```python
from build123d import *

# Parameters (mm, degrees)
F0_W     = 609.6
F0_H     = 304.8
F1_DEPTH = 19.05
F2_W     = 10.795
F2_H     = 52.07
F3_DEPTH = 38.101
F4_W     = 127
F4_H     = 177.8
F5_DEPTH = 6.35


with BuildPart() as f1:
    # F0 (on Top) → F1 (new body, symmetric)
    with BuildSketch(Plane.XY):
        Rectangle(F0_W, F0_H)
    extrude(amount=F1_DEPTH, both=True)

    # F2 (on face) → F3 (cut, through all)
    with BuildSketch(Plane.XY.offset(19.05)):
        with Locations((-152.4, 0)):
            Rectangle(F2_W, F2_H)
        with Locations((152.4, 0)):
            Rectangle(F2_W, F2_H)
    extrude(amount=-F3_DEPTH, mode=Mode.SUBTRACT)

    # F4 (on face) → F5 (cut)
    with BuildSketch(Plane(origin=(0, 0, -19.05), x_dir=(1, 0, 0), z_dir=(0, 0, -1))):
        with Locations((-152.4, 0)):
            Rectangle(F4_W, F4_H)
        with Locations((152.4, 0)):
            Rectangle(F4_W, F4_H)
    extrude(amount=-F5_DEPTH, mode=Mode.SUBTRACT)


solid = f1.part
```
Build history of the part. All positions in model axes, mm. A direction names the side the tool comes from. Give positions to 0.01 mm unless a question says otherwise; leave off trailing zeros. Loops run counter-clockwise (first coordinate to the right, second up) from the corner with the lowest first, then second, coordinate; pieces in that order, holes last.
1) 3-axis set-ups, long thin cutter, end or side, ignore diameter. For faces 4 (the face through (-4, 152.4, 0)), 5 (the face through (-167, -1, -12.7)), 6 (the face through (147.002, 0, 3)): which of +Z, -Z, +X, -X, +Y, -Y reach the whole face in a straight line?
Values follow:
face 4: +Z, -Z, +X, -X, +Y
face 5: -Z
face 6: +Z, -Z
2) Drop a flat-ended pin along its axis: P1, Ø8, axis at x = 211.5, y = -38.5, coming from the -Z side. Give the stop position or say it passes through.
Values follow:
P1: stops at z = -12.7
3) Band-saw the part on A-A on y = 19. List the corners of the cut face in (x, z).
Values follow:
outline: (-304.8, -19.05) - (-215.9, -19.05) - (-215.9, -12.7) - (-157.8, -12.7) - (-157.8, 19.05) - (-304.8, 19.05) - close; (-147, -12.7) - (-88.9, -12.7) - (-88.9, -19.05) - (88.9, -19.05) - (88.9, -12.7) - (147, -12.7) - (147, 19.05) - (-147, 19.05) - close; (157.8, -12.7) - (215.9, -12.7) - (215.9, -19.05) - (304.8, -19.05) - (304.8, 19.05) - (157.8, 19.05) - close
4) Probe line 1 along X through (y, z) = (-7, 9); line 2 along Y through (x, z) = (164, -16.5); line 3 along X through (y, z) = (48, -14). List the from-to ranges inside material, lowest first.
Values follow:
line 1: x = -304.8 to -157.8, -147 to 147, 157.8 to 304.8
line 2: y = -152.4 to -88.9, 88.9 to 152.4
line 3: x = -304.8 to -215.9, -88.9 to 88.9, 215.9 to 304.8
5) Band-saw the part on C-C on x = 177.5. List the corners of the cut face in (y, z), then the cut area to 3 significant figures.
Values follow:
outline: (-152.4, -19.05) - (-88.9, -19.05) - (-88.9, -12.7) - (88.9, -12.7) - (88.9, -19.05) - (152.4, -19.05) - (152.4, 19.05) - (-152.4, 19.05) - close
area: 10,500 mm2
6) Two-plate mould, pull along X, no slides. Class faces 1 (the face through (-4, 2, -19.05)), 2 (the face through (-304.8, -2, 0)), 3 (the face through (-152, -26.035, 3)): released by +X, released by -X, zero draft, split by the parting line, or undercut.
Values follow:
face 1: zero draft
face 2: released by -X
face 3: undercut
7) Band-saw the part on B-B on y = -79.5. List the corners of the cut face in (x, z).
Values follow:
outline: (-304.8, -19.05) - (-215.9, -19.05) - (-215.9, -12.7) - (-88.9, -12.7) - (-88.9, -19.05) - (88.9, -19.05) - (88.9, -12.7) - (215.9, -12.7) - (215.9, -19.05) - (304.8, -19.05) - (304.8, 19.05) - (-304.8, 19.05) - close
